Check sheet for the modelled part. Datum: model origin and axes. Units: mm. Face numbers are marked on the shaded views. Give positions to 0.01 mm unless a question says otherwise; leave off trailing zeros. Write each loop counter-clockwise with the first axis right and the second up, starting at its lowest first coordinate (ties: lowest second). Pieces come first, ordered by that corner, then holes. Notation, with made-up numbers: M -38.5,7.5 L 0.5,7.5 A27 ccw 0.5,46.5 Z; hole C -8,-27 d8. An arc over 180 degrees is marked long. Write item = value, one per line. Start each with the question number.
1) Sectioned sample at C-C, the plane z = 52. Record the cut outline in (x, y).
2) Scan lines: L1, parallel to X at y = 10, z = 0; L2, parallel to Z at x = 38, y = 8.5; L3, parallel to X at y = 2.3, z = 0. Record each from-to range of solid material in increasing order.
3) Sectioned sample at A-A, the plane x = -62. Record the cut outline in (y, z), then the cut area to 3 significant figures.
4) Draft check along Z on the marked faces 1 and 2. Enter one of: pulls with the +Z half, pulls with the -Z half, needs draft (parallel to the pull), parting line crosses it, or undercut.
5) Sectioned sample at B-B, the plane x = 38. Record the cut outline in (y, z).
6) Gauge pin test, flat ends, axial feed: pin 1 (10 mm diameter, centred on x = -44, y = 12.5, fed in from -Z); pin 2 (8 mm diameter, centred on x = 78, y = 11.5, fed in from -Z); pin 3 (6 mm diameter, centred on x = -30.5, z = 28, fed in from +Y). Record the tip position at first contact, or that the pin passes through.
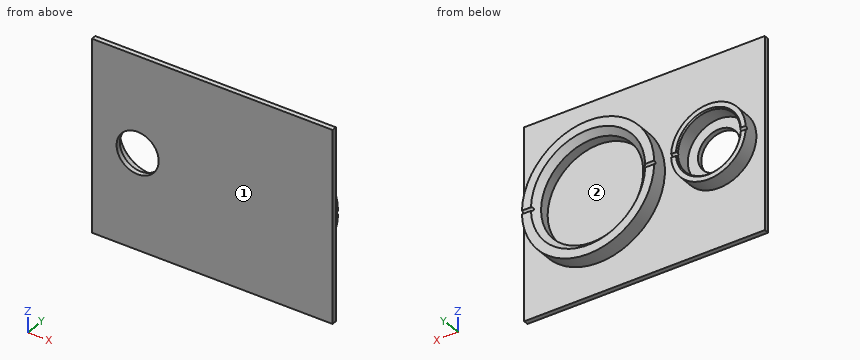
from build123d import *

# Parameters (mm, degrees)
SKETCH1_W                = 200
SKETCH1_H                = 160
BOSS_EXTRUDE1_DEPTH      = 4
SKETCH2_R                = 31
SKETCH2_R_2              = 26
SKETCH2_R_3              = 55
SKETCH2_R_4              = 42.5
BOSS_EXTRUDE2_DEPTH      = 13
CHAMFER2_SIZE            = 5
CHAMFER4_SIZE            = 1
SKETCH9_R                = 17.5
CUT_EXTRUDE8_DEPTH       = 5
SKETCH11_R               = 1.5
CUT_EXTRUDE10_DEPTH      = 101
CUT_EXTRUDE10_DEPTH_BACK = 101


with BuildPart() as part:
    # Sketch1 → Boss-Extrude1 (new body)
    with BuildSketch(Plane(origin=(0, 0, 0), x_dir=(1, 0, 0), z_dir=(0, 1, 0))):
        Rectangle(SKETCH1_W, SKETCH1_H)
    extrude(amount=BOSS_EXTRUDE1_DEPTH)

    # Sketch2 → Boss-Extrude2 (add)
    with BuildSketch(Plane(origin=(0, 4, 0), x_dir=(1, 0, 0), z_dir=(0, 1, 0))):
        with Locations((-62, 0)):
            Circle(SKETCH2_R)
        with Locations((-62, 0)):
            Circle(SKETCH2_R_2, mode=Mode.SUBTRACT)
        with Locations((38, 0)):
            Circle(SKETCH2_R_3)
        with Locations((38, 0)):
            Circle(SKETCH2_R_4, mode=Mode.SUBTRACT)
    extrude(amount=BOSS_EXTRUDE2_DEPTH)

    # Chamfer2
    chamfer2_edges = [part.edges().sort_by_distance(p)[0] for p in [
        (-4.5, 17, 0),
    ]]
    chamfer(chamfer2_edges, length=CHAMFER2_SIZE)

    # Chamfer4
    chamfer4_edges = [part.edges().sort_by_distance(p)[0] for p in [
        (-88, 17, 0),
    ]]
    chamfer(chamfer4_edges, length=CHAMFER4_SIZE)

    # Sketch9 → Cut-Extrude8 (cut, through all)
    with BuildSketch(Plane(origin=(0, 4, 0), x_dir=(1, 0, 0), z_dir=(0, 1, 0))):
        with Locations((-62, 0)):
            Circle(SKETCH9_R)
    extrude(amount=-CUT_EXTRUDE8_DEPTH, mode=Mode.SUBTRACT)

    # Sketch11 → Cut-Extrude10 (cut, two sides)
    with BuildSketch(Plane(origin=(0, 0, 0), x_dir=(0, 0, -1), z_dir=(1, 0, 0))) as cut_extrude10_sk:
        with Locations((0, 17)):
            Circle(SKETCH11_R)
    extrude(amount=CUT_EXTRUDE10_DEPTH, mode=Mode.SUBTRACT)
    extrude(cut_extrude10_sk.sketch, amount=-CUT_EXTRUDE10_DEPTH_BACK, mode=Mode.SUBTRACT)


solid = part.part
Data:
q1.outline = M -100,0 L 100,0 L 100,4 L 55.92,4 L 55.92,17 L 20.08,17 L 20.08,4 L -100,4 Z
q2.L1 = -93 to -88, -36 to -31, -17 to -4.5, 80.5 to 93
q2.L2 = -55 to -42.5, 42.5 to 55
q2.L3 = -100 to -79.5, -44.5 to 100
q3.outline = M 0,-80 L 4,-80 L 4,-31 L 17,-31 L 17,-27 L 16,-26 L 4,-26 L 4,-17.5 L 0,-17.5 Z; M 0,17.5 L 4,17.5 L 4,26 L 16,26 L 17,27 L 17,31 L 4,31 L 4,80 L 0,80 Z
q3.area = 629 mm2
q4.face_1 = needs draft
q4.face_2 = undercut
q5.outline = M 0,-80 L 4,-80 L 4,-55 L 17,-55 L 17,-47.5 L 12,-42.5 L 4,-42.5 L 4,42.5 L 12,42.5 L 17,47.5 L 17,55 L 4,55 L 4,80 L 0,80 Z
q6.pin_1 = -28.14
q6.pin_2 = -41.58
q6.pin_3 = 4
